Work out the finished part from the listing and answer in its coordinate system (mm). A direction names the side the tool comes from. Coordinates: 2 decimals unless noted, no trailing zeros. Order: outer loops, then holes, each group sorted by start corner. A loop starts at its lowest first (then second) coordinate and runs counter-clockwise, first axis right, second up.
1. A tool of negligible diameter and unlimited length cuts with its end or side. For faces 4 (the flat face through (6.4, 13.42, -10.74)), 5 (the flat face through (-4, 8, 10)), 6 (the cylindrical face through (11.36, 21.797, -0.039)), 7 (the flat face through (2, 23, 8)), 8 (the cylindrical face through (-11.298, 21.859, 0.039)), from which of +Z, -Z, +X, -X, +Y, -Y can it reach the whole face along a straight path? Write none if from no direction.
2. The part is cut by section B-B, the plane y = 3.5. Give the vertices of the cut face in (x, z), then the cut area to 3 significant figures.
3. Determine the mould class of faces 1 (the cylindrical face through (-5.62, 21.86, 9.8)), 2 (the cylindrical face through (-7.81, 11.34, 1.73)), 3 (the flat face through (-6.1, 13.42, -10.91)) for opening direction Z: +Z half, -Z half, draft (parallel to the pull), parting line (faces both ways), or undercut.
4. Flat-ended cylindrical pins translate along their axes: pin 1 Ø1 at (x, y) = (-9.5, 14) entering from +Z; pin 2 Ø3 at (x, y) = (1.5, 2.5) entering from -Z; pin 3 Ø5 at (y, z) = (19.5, 10.5) entering from -X. Find the tip coordinate at first contact, or state that the pin passes through.
5. The part is cut by section A-A, the plane y = 10.75. Give the vertices of the cut face in (x, z).
6. Find the intervals of material crossed by probe 1 along X at (y, z) = (7, 0); probe 2 along Z at (x, y) = (1.5, 20.5); probe 3 along Z at (x, y) = (2, 5), in increasing order.
```python
from build123d import *

# Parameters (mm, degrees)
SKETCH1_R           = 10
BOSS_EXTRUDE1_DEPTH = 8
BOSS_EXTRUDE2_DEPTH = 15
CUT_EXTRUDE1_REACH  = 31.909
SKETCH3_R           = 8
FILLET1_R           = 4


with BuildPart() as part:
    # Sketch1 → Boss-Extrude1 (new body)
    with BuildSketch(Plane(origin=(0, 0, 0), x_dir=(1, 0, 0), z_dir=(0, 1, 0))):
        with Locations(Location((0, 0, 0), (0, 0, 270))):
            Circle(SKETCH1_R)
    extrude(amount=BOSS_EXTRUDE1_DEPTH)

    # Sketch2 → Boss-Extrude2 (add)
    with BuildSketch(Plane(origin=(0, 8, 0), x_dir=(1, 0, 0), z_dir=(0, 1, 0))):
        Polygon((12.460098185, -7.285553277), (12.539523311, 7.147984923), (0.079425127, 14.4335382), (-12.460098185, 7.285553277), (-12.539523311, -7.147984923), (-0.079425127, -14.4335382), align=None)
    extrude(amount=BOSS_EXTRUDE2_DEPTH)

    # Sketch3 → Cut-Extrude1 (cut, up to next)
    with BuildSketch(Plane.XZ, mode=Mode.PRIVATE) as cut_extrude1_sk1:
        with Locations(Location((0, 0, 0), (0, 0, 270))):
            Circle(SKETCH3_R)
    cut_extrude1_tool1 = extrude(cut_extrude1_sk1.sketch, amount=-CUT_EXTRUDE1_REACH, mode=Mode.PRIVATE) & part.part
    add(cut_extrude1_tool1.solids().sort_by_distance((0, 0, 0))[0], mode=Mode.SUBTRACT)

    # Fillet1
    fillet1_edges = [part.edges().sort_by_distance(p)[0] for p in [
        (6.190336529, 23, 10.859545739),
        (12.499810748, 23, 0.068784177),
        (6.309474219, 23, -10.790761562),
        (-6.190336529, 23, -10.859545739),
        (-12.499810748, 23, -0.068784177),
        (-6.309474219, 23, 10.790761562),
    ]]
    fillet(fillet1_edges, radius=FILLET1_R)


solid = part.part
```
Geometry says:
1. face 4: -Z, +X, +Y, -Y
1. face 5: -Y
1. face 6: +Z, +X, +Y
1. face 7: +Z, -Z, +X, -X, +Y
1. face 8: -Z, -X, +Y
2. outline: circle Ø20 at (0, 0); hole circle Ø16 at (0, 0)
2. area: 113 mm2
3. face 1: +Z half
3. face 2: undercut
3. face 3: -Z half
4. pin 1: stops at z = 9.22
4. pin 2: stops at z = -10
4. pin 3: stops at x = -11.05
5. outline: (-12.54, 7.15) - (-12.46, -7.29) - (0.08, -14.43) - (12.54, -7.15) - (12.46, 7.29) - (-0.08, 14.43) - close; hole circle Ø16 at (0, 0)
6. probe 1: x = -10 to -8, 8 to 10
6. probe 2: z = -13.26 to -7.86, 7.86 to 13.2
6. probe 3: z = -9.8 to -7.75, 7.75 to 9.8
